```python
from build123d import *

# Parameters (mm, degrees)
F0_W     = 37.5
F0_H     = 62.5
F1_DEPTH = 26
F2_R     = 44.5
F2_W     = 37.5
F2_H     = 62.5
F3_DEPTH = 20
F4_T     = -2


with BuildPart() as f1:
    # F0 (on Front) → F1 (new body)
    with BuildSketch(Plane.XZ):
        with Locations((-18.75, 31.25)):
            Rectangle(F0_W, F0_H)
    extrude(amount=F1_DEPTH)

    # F2 (on face) → F3 (join)
    with BuildSketch(Plane.XZ.offset(26)):
        with Locations((-18.75, 31.25)):
            Circle(F2_R)
        with Locations((-18.75, 31.25)):
            Rectangle(F2_W, F2_H, mode=Mode.SUBTRACT)
        with Locations((-18.75, 31.25)):
            Rectangle(F2_W, F2_H)
    extrude(amount=F3_DEPTH)

    # F4
    f4_openings = [f1.faces().sort_by_distance(p)[0] for p in [
        (-18.75, -46, 31.25),
        (-18.75, 0, 31.25),
    ]]
    offset(amount=F4_T, openings=f4_openings, kind=Kind.INTERSECTION)


solid = f1.part
```
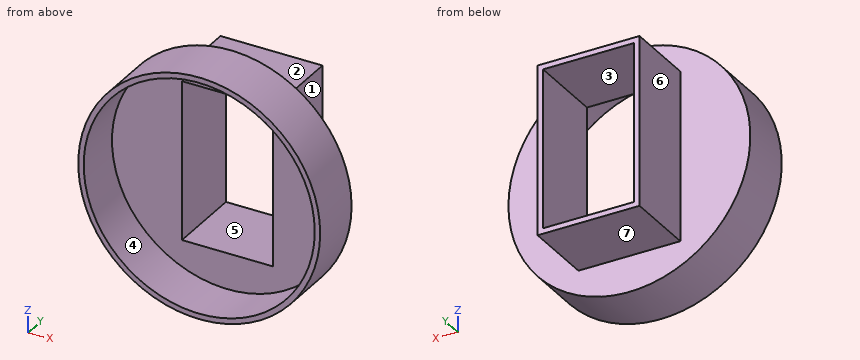
Design review of the part built by this model. Coordinates are the model's own, in mm. Face numbers are marked on the shaded views. A direction names the side the tool comes from. Give positions to 0.01 mm unless a question says otherwise; leave off trailing zeros. Write each loop counter-clockwise with the first axis right and the second up, starting at its lowest first coordinate (ties: lowest second). Pieces come first, ordered by that corner, then holes. Notation, with made-up numbers: (15, -17.5) - (44, -17.5) arc R26 ccw to (44, 11.5) - close; hole circle Ø5 at (-29, 76). An arc over 180 degrees is marked (long way). Return JSON: item names as keys, results as strings. Group by question number.
(1) We need section C-C, the plane x = -18.75. Give the boundary of the cut face in (y, z).
(2) Insertion check: pin 1 (12 mm diameter, centred on y = -36, z = -1.5, fed in from -X); pin 2 (1 mm diameter, centred on x = -6.5, z = -2, fed in from +Y); pin 3 (12 mm diameter, centred on y = -32.5, z = 20, fed in from +X); pin 4 (12 mm diameter, centred on x = -2.5, z = 65, fed in from -Y). Each pin has a flat end and moves straight along its axis. Give the tip position at first contact, or say it passes through.
(3) We need section A-A, the plane y = -21. Give the boundary of the cut face in (x, z), then the cut area to 3 significant figures.
(4) To check wall thickness, follow probe 1 along X at (y, z) = (-4, 60); probe 2 along Z at (x, y) = (-25.5, -25); probe 3 along Z at (x, y) = (-18.75, -42). State the ranges of each line that lie inside material, in increasing order.
(5) We need section B-B, the plane z = 31.25. Give the boundary of the cut face in (x, y).
(6) Machinability: for the marked faces 1, 2, 3 and 4, which of the approach directions +Z, -Z, +X, -X, +Y, -Y give a long, thin tool a straight path to every point of the face, cutting with its end or side? Answer none if there is none.
(7) Mouldability with a two-part tool opening along Z and no side actions: class the marked faces 5, 6 and 7 as +Z half, -Z half, draft (parallel to the pull), parting line (faces both ways), or undercut.
(8) We need section D-D, the plane x = -50.5. Give the boundary of the cut face in (y, z), then the cut area to 3 significant figures.
Reported:
{
 "1": {"outline": "(-46, -13.25) - (-26, -13.25) - (-26, 0) - (0, 0) - (0, 2) - (-28, 2) - (-28, -11.25) - (-46, -11.25) - close; (-46, 73.75) - (-28, 73.75) - (-28, 60.5) - (0, 60.5) - (0, 62.5) - (-26, 62.5) - (-26, 75.75) - (-46, 75.75) - close"},
 "2": {"pin 1": "stops at x = -54.31", "pin 2": "stops at y = -26", "pin 3": "stops at x = 25.44", "pin 4": "stops at y = -46"},
 "3": {"outline": "(-37.5, 0) - (0, 0) - (0, 62.5) - (-37.5, 62.5) - close; hole (-35.5, 2) - (-2, 2) - (-2, 60.5) - (-35.5, 60.5) - close", "area": "384 mm2"},
 "4": {"probe 1": "x = -37.5 to -35.5, -2 to 0", "probe 2": "z = 0 to 2, 60.5 to 62.5", "probe 3": "z = -13.25 to -11.25, 73.75 to 75.75"},
 "5": {"outline": "(-63.25, -46) - (-61.25, -46) - (-61.25, -28) - (-35.5, -28) - (-35.5, 0) - (-37.5, 0) - (-37.5, -26) - (-63.25, -26) - close; (-2, -28) - (23.75, -28) - (23.75, -46) - (25.75, -46) - (25.75, -26) - (0, -26) - (0, 0) - (-2, 0) - close"},
 "6": {"face 1": "+Z, -Z, +X, +Y", "face 2": "+Z, +X, -X, +Y", "face 3": "+Y, -Y", "face 4": "-Y"},
 "7": {"face 5": "undercut", "face 6": "draft", "face 7": "-Z half"},
 "8": {"outline": "(-46, 0.07) - (-26, 0.07) - (-26, 62.43) - (-46, 62.43) - (-46, 59.5) - (-28, 59.5) - (-28, 3) - (-46, 3) - close", "area": "230 mm2"}
}
